Read the model definition and answer for the solid it produces. Units are mm, in the model's axes. Face numbers are marked on the shaded views. A direction names the side the tool comes from. Give positions to 0.01 mm unless a question says otherwise; leave off trailing zeros. Write each loop counter-clockwise with the first axis right and the second up, starting at its lowest first coordinate (ties: lowest second). Pieces come first, ordered by that corner, then holes. Notation, with made-up numbers: M 87,21.5 L 117,21.5 A29 ccw 117,50.5 Z; hole C -15,83 d1. An arc over 180 degrees is marked long. Use a Markdown table: item, result. Add a question column.
Item 1: Consider probe 1 along X at (y, z) = (14.25, 1); probe 2 along X at (y, z) = (7, 15); probe 3 along Z at (x, y) = (-73, 2.75). Determine where each line is inside the solid, lowest interval first. Write a range as [from, to].
Item 2: A cutting plane is placed at D-D on z = 14. Determine the outline of the cut face in (x, y).
Item 3: Given P1, Ø5, axis at x = -9, y = 10.5, coming from the -Z side; P2, Ø7.5, axis at x = -51.5, y = 5, coming from the +Z side; P3, Ø4, axis at x = -2.5, z = 16, coming from the +Y side; P4, Ø5, axis at y = 12.5, z = -6, coming from the +X side, each flat-ended and moving along its own axis, determine where each tip first touches the part or whether it passes through.
Item 4: A cutting plane is placed at C-C on x = -58. Determine the outline of the cut face in (y, z), then the cut area to 4 significant figures.
Item 5: For the marked faces 4, 5 and 6, determine the directions among +Z, -Z, +X, -X, +Y, -Y from which every point of the face is accessible in a straight line to the end or side of a thin tool.
Item 6: A cutting plane is placed at B-B on y = 8. Determine the outline of the cut face in (x, z), then the cut area to 3 significant figures.
Item 7: A cutting plane is placed at A-A on z = 4. Determine the outline of the cut face in (x, y), then the cut area to 3 significant figures.
Item 8: The mould has two halves that part along X. Classify the marked faces 1, 2 and 3: pulls with the +X half, pulls with the -X half, needs draft (parallel to the pull), parting line crosses it, or undercut.
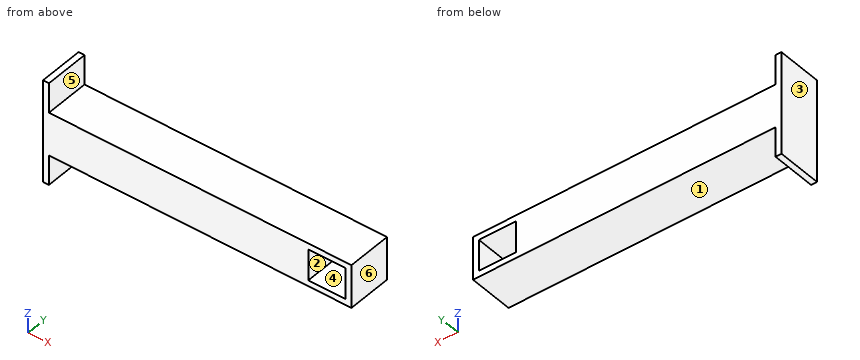
from build123d import *

# Parameters (mm, degrees)
SKETCH1_W           = 12.5
SKETCH1_H           = 10.5
BOSS_EXTRUDE2_DEPTH = 15


with BuildPart() as part:
    # Sketch1 → Boss-Extrude2 (new body)
    with BuildSketch(Plane(origin=(0, 0, 0), x_dir=(1, 0, 0), z_dir=(0, 1, 0))):
        Polygon((-87.25, -22.5), (-87.25, -12.5), (-2, -12.5), (14.5, -12.5), (14.5, 2), (-2, 2), (-87.25, 2), (-87.25, 12), (-89.25, 12), (-89.25, -22.5), align=None)
        with Locations((6.25, -5.25)):
            Rectangle(SKETCH1_W, SKETCH1_H, mode=Mode.SUBTRACT)
    extrude(amount=BOSS_EXTRUDE2_DEPTH)


solid = part.part
Filled in:
| question | item | result |
|---|---|---|
| 1 | probe 1 | [-89.25, 0], [12.5, 14.5] |
| 1 | probe 2 | [-89.25, -87.25] |
| 1 | probe 3 | [-2, 12.5] |
| 2 | outline | M -89.25,0 L -87.25,0 L -87.25,15 L -89.25,15 Z |
| 3 | P1 | z = -2 |
| 3 | P2 | z = 12.5 |
| 3 | P3 | through |
| 3 | P4 | x = -87.25 |
| 4 | outline | M 0,-2 L 15,-2 L 15,12.5 L 0,12.5 Z |
| 4 | area | 217.5 mm² |
| 5 | face 4 | +Y, -Y |
| 5 | face 5 | +Z, +X, +Y, -Y |
| 5 | face 6 | +Z, -Z, +X, +Y, -Y |
| 6 | outline | M -89.25,-12 L -87.25,-12 L -87.25,-2 L 14.5,-2 L 14.5,12.5 L -87.25,12.5 L -87.25,22.5 L -89.25,22.5 Z; hole M 0,0 L 12.5,0 L 12.5,10.5 L 0,10.5 Z |
| 6 | area | 1,410 mm² |
| 7 | outline | M -89.25,0 L 0,0 L 0,15 L -89.25,15 Z; M 12.5,0 L 14.5,0 L 14.5,15 L 12.5,15 Z |
| 7 | area | 1,370 mm² |
| 8 | face 1 | needs draft |
| 8 | face 2 | undercut |
| 8 | face 3 | pulls with the -X half |
